Part model, mm, in its own coordinate system. Face numbers are marked on the shaded views. Coordinates: 2 decimals unless noted, no trailing zeros. Write each loop counter-clockwise with the first axis right and the second up, starting at its lowest first coordinate (ties: lowest second). Pieces come first, ordered by that corner, then holes. Notation, with made-up numbers: (-36, -37.75) - (21, -37.75) arc R18 ccw to (21, -33.75) - close; hole circle Ø10 at (74.5, 69). An arc over 180 degrees is marked (long way). Use a Markdown table: item, result.
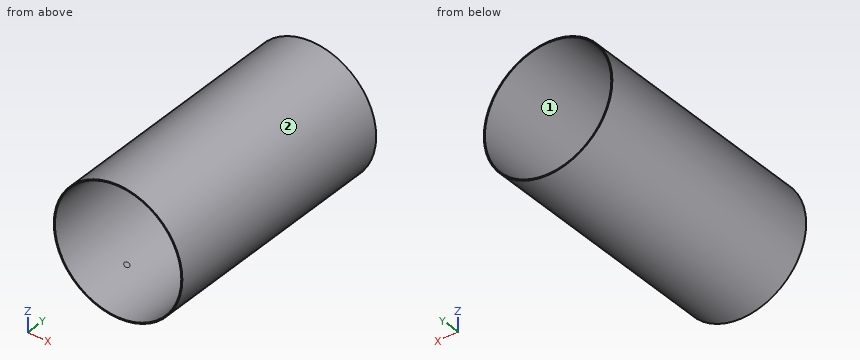
```python
from build123d import *

# Parameters (mm, degrees)
SKETCH1_R           = 77.724
SKETCH1_R_2         = 76.454
EXTRUDE_THIN2_DEPTH = 304.8
SKETCH3_R           = 3.302
CUT_EXTRUDE2_DEPTH  = 2.54
CIRPATTERN2_COUNT   = 3


with BuildPart() as part:
    # Sketch1 → Extrude-Thin2 (new body)
    with BuildSketch(Plane(origin=(0, 0, 0), x_dir=(1, 0, 0), z_dir=(0, 1, 0))):
        Circle(SKETCH1_R)
        Circle(SKETCH1_R_2, mode=Mode.SUBTRACT)
    extrude(amount=EXTRUDE_THIN2_DEPTH)

    # Sketch3 → Cut-Extrude2 (cut)
    with BuildSketch(Plane.ZY.offset(-76.454)):
        with Locations((0, 63.5)):
            Circle(SKETCH3_R)
    cut_extrude2 = extrude(amount=CUT_EXTRUDE2_DEPTH, mode=Mode.SUBTRACT)

    # CirPattern2: Cut-Extrude2 ×3 about axis
    cirpattern2_axis = Axis((0, 0, 0), (0, 1, 0))
    for i in range(1, CIRPATTERN2_COUNT):
        add(cut_extrude2.rotate(cirpattern2_axis, i * 360 / CIRPATTERN2_COUNT), mode=Mode.SUBTRACT)


solid = part.part
```
Item 1: Drop flat-ended pins along their axis: P1, Ø1, axis at x = 4.5, y = 166, coming from the +Z side; P2, Ø10, axis at x = -24.5, y = 209, coming from the +Z side; P3, Ø6, axis at y = 183.5, z = 34.5, coming from the -X side. Give the stop position or say it passes through.
From the geometry:
| item | result |
|---|---|
| P1 | z = 77.62 |
| P2 | z = 75.24 |
| P3 | x = -71.05 |
Item 2: Drill centre lines: probe 1 along Z at (x, y) = (0, 234); probe 2 along X at (y, z) = (88.5, -30). Where is each one in solid material? Low to high.
From the geometry:
| item | result |
|---|---|
| probe 1 | -77.72 to -76.45, 76.45 to 77.72 |
| probe 2 | -71.7 to -70.32, 70.32 to 71.7 |
Item 3: Band-saw the part on A-A, the plane x = 0. Give the cut face in (y, z).
From the geometry:
| item | result |
|---|---|
| outline | (0, -77.72) - (304.8, -77.72) - (304.8, -76.45) - (0, -76.45) - close; (0, 76.45) - (304.8, 76.45) - (304.8, 77.72) - (0, 77.72) - close |
Item 4: Band-saw the part on C-C, the plane y = 63.5. Give the cut face in (x, z), then the cut area to 3 significant figures.
From the geometry:
| item | result |
|---|---|
| outline | circle Ø155.45 at (0, 0); hole (-41.09, -64.56) - (-35.37, -67.86) - (-35.33, -67.8) arc R76.45 ccw to (76.38, -3.3) - (76.45, -3.3) - (76.45, 3.3) - (76.38, 3.3) arc R76.45 ccw to (-35.33, 67.8) - (-35.37, 67.86) - (-41.09, 64.56) - (-41.05, 64.5) arc R76.45 ccw to (-41.05, -64.5) - close |
| area | 615 mm^2 |
Item 5: Two-plate mould, pull along Z, no slides. Class the marked faces 1 and 2: pulls with the +Z half, pulls with the -Z half, needs draft (parallel to the pull), parting line crosses it, or undercut.
From the geometry:
| item | result |
|---|---|
| face 1 | undercut |
| face 2 | parting line crosses it |
Item 6: Band-saw the part on D-D, the plane y = 249.5. Give the cut face in (x, z), then the cut area to 3 significant figures.
From the geometry:
| item | result |
|---|---|
| outline | circle Ø155.45 at (0, 0); hole circle Ø152.91 at (0, 0) |
| area | 615 mm^2 |
